Model file for the job. Use its own axes, mm. A direction names the side the tool comes from. Coordinates: 2 decimals unless noted, no trailing zeros. Loops run counter-clockwise (first coordinate to the right, second up) from the corner with the lowest first, then second, coordinate; pieces in that order, holes last.
from build123d import *

# Parameters (mm, degrees)
SKETCH1_W           = 203.2
SKETCH1_H           = 33.02
BOSS_EXTRUDE1_DEPTH = 50.8
SKETCH4_W           = 75.174345078
SKETCH4_H           = 39.769068734
CUT_EXTRUDE2_DEPTH  = 119.294211186
SKETCH5_W           = 75.174345078
SKETCH5_H           = 9.289068734
BOSS_EXTRUDE3_DEPTH = 20.32
BOSS_EXTRUDE4_START = 15.24
SKETCH6_R           = 2.5
BOSS_EXTRUDE4_DEPTH = 1.27
BOSS_EXTRUDE5_START = -15.24
SKETCH6_3_R         = 2.5
BOSS_EXTRUDE5_DEPTH = 1.27


with BuildPart() as part:
    # Sketch1 → Boss-Extrude1 (new body)
    with BuildSketch(Plane(origin=(0, 0, 0), x_dir=(1, 0, 0), z_dir=(0, 1, 0))):
        Rectangle(SKETCH1_W, SKETCH1_H)
    extrude(amount=BOSS_EXTRUDE1_DEPTH)

    # Sketch4 → Cut-Extrude2 (cut, through all)
    with BuildSketch(Plane.XY.offset(16.51)):
        with Locations((-64.012827461, 30.915465633)):
            Rectangle(SKETCH4_W, SKETCH4_H)
    extrude(amount=-CUT_EXTRUDE2_DEPTH, mode=Mode.SUBTRACT)

    # Sketch5 → Boss-Extrude3 (add)
    with BuildSketch(Plane.XY.offset(16.51)):
        with Locations((-64.012827461, 15.675465633)):
            Rectangle(SKETCH5_W, SKETCH5_H)
    extrude(amount=-BOSS_EXTRUDE3_DEPTH)

    # Sketch6 → Boss-Extrude4 (add, symmetric)
    # profile 1 of 2: a face of its own
    with BuildSketch(Plane.XY.offset(BOSS_EXTRUDE4_START)):
        Polygon((4.572, 50.8), (-4.572, 50.8), (-26.425654922, 50.8), (-26.425654922, 20.32), (-101.6, 20.32), (-101.6, 0), (101.6, 0), (101.6, 50.8), align=None)
    # profile 2 of 2: a face of its own
    with BuildSketch(Plane.XY.offset(BOSS_EXTRUDE4_START)):
        with BuildLine():
            Line((-4.572, 66.294), (-4.572, 50.8))
            Line((-4.572, 50.8), (4.572, 50.8))
            Line((4.572, 50.8), (4.572, 66.294))
            ThreePointArc((4.572, 66.294), (0, 70.866), (-4.572, 66.294))
        make_face()
        with Locations((0, 66.294)):
            Circle(SKETCH6_R, mode=Mode.SUBTRACT)
    extrude(amount=BOSS_EXTRUDE4_DEPTH, both=True)

    # Sketch6_3 → Boss-Extrude5 (add, symmetric)
    with BuildSketch(Plane.XY.offset(BOSS_EXTRUDE5_START)):
        with BuildLine():
            Line((-4.572, 50.8), (-4.572, 66.294))
            ThreePointArc((-4.572, 66.294), (0, 70.866), (4.572, 66.294))
            Line((4.572, 66.294), (4.572, 50.8))
            Line((4.572, 50.8), (-4.572, 50.8))
        make_face()
        with Locations((0, 66.294)):
            Circle(SKETCH6_3_R, mode=Mode.SUBTRACT)
    extrude(amount=BOSS_EXTRUDE5_DEPTH, both=True)


solid = part.part
Q1. Mould opens along X. For faces 1 (the cylindrical face through (0.101, 70.865, 15.258)), 2 (the flat face through (-65, 16, -3.81)), 3 (the cylindrical face through (-0.542, 63.853, -15.258)) say: +X half, -X half, draft (parallel to the pull), parting line (faces both ways), or undercut.
Answers:
face 1: parting line
face 2: draft
face 3: undercut
Q2. Slice it at C-C (y = 15). List the corners of the cut face in (x, z), and give its area (3 significant figures).
Answers:
outline: (-101.6, -3.81) - (-26.43, -3.81) - (-26.43, -16.51) - (101.6, -16.51) - (101.6, 16.51) - (-101.6, 16.51) - close
area: 5,750 mm2
Q3. Drill centre lines: line 1 (Y direction, x = 0, z = 15.15); line 2 (X direction, y = 17.5, z = -10); line 3 (Y direction, x = 79, z = -12). Where is each one in solid material? Low to high.
Answers:
line 1: y = 0 to 63.79, 68.79 to 70.87
line 2: x = -26.43 to 101.6
line 3: y = 0 to 50.8
Q4. Slice it at D-D (z = -0.5). List the corners of the cut face in (x, y).
Answers:
outline: (-101.6, 0) - (101.6, 0) - (101.6, 50.8) - (-26.43, 50.8) - (-26.43, 20.32) - (-101.6, 20.32) - close
Q5. Slice it at B-B (x = 0). List the corners of the cut face in (y, z), and give its area (3 significant figures).
Answers:
outline: (0, -16.51) - (63.79, -16.51) - (63.79, -13.97) - (50.8, -13.97) - (50.8, 13.97) - (63.79, 13.97) - (63.79, 16.51) - (0, 16.51) - close; (68.79, -16.51) - (70.87, -16.51) - (70.87, -13.97) - (68.79, -13.97) - close; (68.79, 13.97) - (70.87, 13.97) - (70.87, 16.51) - (68.79, 16.51) - close
area: 1,750 mm2
Q6. Flat gauge pins, fed straight in: P1, Ø0.8, axis at y = 61, z = 16, coming from the -X side; P2, Ø1, axis at x = 47.5, z = 13, coming from the -Y side; P3, Ø4, axis at x = -75, z = -8.5, coming from the +Y side; P4, Ø3, axis at y = 60.5, z = 16, coming from the +X side. Where does each tip first touch, or does it go through?
Answers:
P1: stops at x = -4.57
P2: stops at y = 0
P3: stops at y = 11.03
P4: stops at x = 4.57
Q7. Slice it at A-A (y = 54). List the corners of the cut face in (x, z).
Answers:
outline: (-4.57, -16.51) - (4.57, -16.51) - (4.57, -13.97) - (-4.57, -13.97) - close; (-4.57, 13.97) - (4.57, 13.97) - (4.57, 16.51) - (-4.57, 16.51) - close
Q8. Which spindle directions (+Z, -Z, +X, -X, +Y, -Y) get a long thin tool onto all of the face, cutting with end or side? Do faces 4 (the flat face through (0, 59, 13.97)), 5 (the flat face through (-65, 11.031, -10)), 6 (the flat face through (-65, 20.32, 6)). Say none if no direction does.
Answers:
face 4: +X, -X, +Y
face 5: -Z, -X, +Y
face 6: +Z, -Z, -X, +Y
